Geometry: final body of the model. Coordinates: model frame, mm. Give positions to 0.01 mm unless a question says otherwise; leave off trailing zeros. Write each loop counter-clockwise with the first axis right and the second up, starting at its lowest first coordinate (ties: lowest second). Pieces come first, ordered by that corner, then holes. Notation, with made-up numbers: M 81,87 L 91,87 A25 cw 91,105 Z; hole C 80.5,88.25 d10. An arc over 180 degrees is marked long. Answer as a JSON object with one key per item and string values.
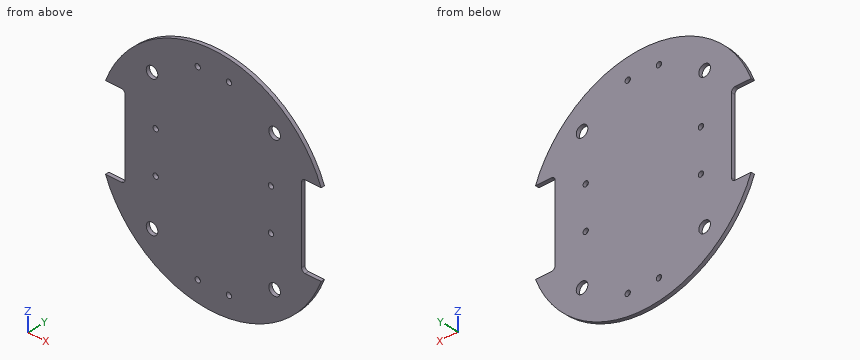
from build123d import *

# Parameters (mm, degrees)
SKETCH1_R               = 49.78
EXTRUDE1_DEPTH          = 1.5875
SKETCH2_R               = 2.5
EXTRUDE2_DEPTH          = 10
CUT_EXTRUDE1_DEPTH      = 71.417447811
FILLET5_R               = 1.6
FILLET5_OF_MIRROR4_R    = 1.6
SKETCH4_R               = 1.145
CUT_EXTRUDE2_DEPTH      = 69.130587523
MIRROR7_COPY_1_SKETCH_R = 1.145
MIRROR7_COPY_1_DEPTH    = 69.130587523
SKETCH6_R               = 1.143
CUT_EXTRUDE4_DEPTH      = 69.130587523
MIRROR9_COPY_1_SKETCH_R = 1.143
MIRROR9_COPY_1_DEPTH    = 69.130587523


with BuildPart() as part:
    # Sketch1 → Extrude1 (new body)
    with BuildSketch(Plane(origin=(0, 0, 0), x_dir=(1, 0, 0), z_dir=(0, 1, 0))):
        with Locations(Location((0, 0, 0), (0, 0, 270))):
            Circle(SKETCH1_R)
    extrude(amount=EXTRUDE1_DEPTH)

    # Sketch2 → Extrude2 (cut)
    with BuildSketch(Plane(origin=(0, 1.5875, 0), x_dir=(-1, 0, 0), z_dir=(0, 1, 0))):
        with Locations(Location((-26.42, -29.72, 0), (0, 0, 90))):
            Circle(SKETCH2_R)
        with Locations(Location((-26.42, 29.72, 0), (0, 0, 90))):
            Circle(SKETCH2_R)
    extrude2 = extrude(amount=-EXTRUDE2_DEPTH, mode=Mode.SUBTRACT)

    # Sketch3 → Cut-Extrude1 (cut, through all)
    with BuildSketch(Plane(origin=(0, 1.5875, 0), x_dir=(1, 0, 0), z_dir=(0, 1, 0))):
        with BuildLine():
            Line((38.03, 0), (38.03, 17.8))
            Line((38.03, 17.8), (46.488798651, 17.8))
            ThreePointArc((46.488798651, 17.8), (49.78, 0), (46.488798651, -17.8))
            Line((46.488798651, -17.8), (38.03, -17.8))
            Line((38.03, -17.8), (38.03, 0))
        make_face()
    cut_extrude1 = extrude(amount=-CUT_EXTRUDE1_DEPTH, mode=Mode.SUBTRACT)

    # Fillet5
    fillet5_edges = [part.edges().sort_by_distance(p)[0] for p in [
        (38.03, 0.79375, 17.8),
        (38.03, 0.79375, -17.8),
    ]]
    fillet(fillet5_edges, radius=FILLET5_R)

    # Mirror4: Cut-Extrude1 across plane
    add(cut_extrude1.mirror(Plane(origin=(0, 0, 0), x_dir=(0, 0, 1), z_dir=(1, 0, 0))), mode=Mode.SUBTRACT)

    # Fillet5 of Mirror4
    fillet5_of_mirror4_edges = [part.edges().sort_by_distance(p)[0] for p in [
        (-38.03, 0.79375, 17.8),
        (-38.03, 0.79375, -17.8),
    ]]
    fillet(fillet5_of_mirror4_edges, radius=FILLET5_OF_MIRROR4_R)

    # Sketch4 → Cut-Extrude2 (cut, through all)
    with BuildSketch(Plane(origin=(0, 1.5875, 0), x_dir=(1, 0, 0), z_dir=(0, 1, 0))):
        with Locations(Location((6.73, 40.5, 0), (0, 0, 270))):
            Circle(SKETCH4_R)
    cut_extrude2 = extrude(amount=-CUT_EXTRUDE2_DEPTH, mode=Mode.SUBTRACT)

    # Mirror5: Cut-Extrude2 across plane
    add(cut_extrude2.mirror(Plane(origin=(0, 0, 0), x_dir=(0, 0, 1), z_dir=(1, 0, 0))), mode=Mode.SUBTRACT)

    # Mirror7: Cut-Extrude2 across plane
    add(cut_extrude2.mirror(Plane.XY), mode=Mode.SUBTRACT)

    # Mirror7 copy 1 sketch → Mirror7 copy 1 (cut, through all)
    with BuildSketch(Plane(origin=(0, 1.5875, 0), x_dir=(-1, 0, 0), z_dir=(0, 1, 0))):
        with Locations(Location((6.73, 40.5, 0), (0, 0, 270))):
            Circle(MIRROR7_COPY_1_SKETCH_R)
    extrude(amount=-MIRROR7_COPY_1_DEPTH, mode=Mode.SUBTRACT)

    # Mirror1: Extrude2 across plane
    add(extrude2.mirror(Plane(origin=(0, 0, 0), x_dir=(0, 0, 1), z_dir=(1, 0, 0))), mode=Mode.SUBTRACT)

    # Sketch6 → Cut-Extrude4 (cut, through all)
    with BuildSketch(Plane(origin=(0, 1.5875, 0), x_dir=(1, 0, 0), z_dir=(0, 1, 0))):
        with Locations(Location((24.83, 9, 0), (0, 0, 270))):
            Circle(SKETCH6_R)
    cut_extrude4 = extrude(amount=-CUT_EXTRUDE4_DEPTH, mode=Mode.SUBTRACT)

    # Mirror8: Cut-Extrude4 across plane
    add(cut_extrude4.mirror(Plane.XY), mode=Mode.SUBTRACT)

    # Mirror9: Cut-Extrude4 across plane
    add(cut_extrude4.mirror(Plane(origin=(0, 0, 0), x_dir=(0, 0, 1), z_dir=(1, 0, 0))), mode=Mode.SUBTRACT)

    # Mirror9 copy 1 sketch → Mirror9 copy 1 (cut, through all)
    with BuildSketch(Plane(origin=(0, 1.5875, 0), x_dir=(-1, 0, 0), z_dir=(0, 1, 0))):
        with Locations(Location((24.83, 9, 0), (0, 0, 270))):
            Circle(MIRROR9_COPY_1_SKETCH_R)
    extrude(amount=-MIRROR9_COPY_1_DEPTH, mode=Mode.SUBTRACT)


solid = part.part
1) Line query: line 1 (X direction, y = 0.5, z = -40.5) (3 decimals); line 2 (X direction, y = 1.5, z = 39.5); line 3 (Z direction, x = -24.83, y = 1.1). Output: solid intervals per line, ascending. Write a range as from..to.
Geometry check:
{"line 1": "x = -28.945..-7.875, -5.585..5.585, 7.875..28.945", "line 2": "x = -30.3..-7.29, -6.17..6.17, 7.29..30.3", "line 3": "z = -43.15..-31.65, -27.79..-10.14, -7.86..7.86, 10.14..27.79, 31.65..43.15"}
2) Contact query for a flat-ended pin moving along its axis: P1, Ø6, axis at x = -26.42, z = 29.72, coming from the -Y side. Output: stop coordinate, or through.
Geometry check:
{"P1": "stops at y = 0"}
3) Cut plane D-D on z = -2. Return loops of the section in (x, y).
Geometry check:
{"outline": "M -38.03,0 L 38.03,0 L 38.03,1.59 L -38.03,1.59 Z"}
4) Cut plane C-C on x = 6.73. Return loops of the section in (y, z) (1 decimal).
Geometry check:
{"outline": "M 0,-49.3 L 1.6,-49.3 L 1.6,-41.6 L 0,-41.6 Z; M 0,-39.4 L 1.6,-39.4 L 1.6,39.4 L 0,39.4 Z; M 0,41.6 L 1.6,41.6 L 1.6,49.3 L 0,49.3 Z"}
5) Cut plane B-B on z = -29.72. Return loops of the section in (x, y), and give its area (3 significant figures).
Geometry check:
{"outline": "M -39.93,0 L -28.92,0 L -28.92,1.59 L -39.93,1.59 Z; M -23.92,0 L 23.92,0 L 23.92,1.59 L -23.92,1.59 Z; M 28.92,0 L 39.93,0 L 39.93,1.59 L 28.92,1.59 Z", "area": "111 mm2"}
6) Cut plane A-A on y = 0.45. Give the number of separate pieces and of enclosed holes in the cut face, and give its area (3 significant figures).
Geometry check:
{"separate pieces": "1", "enclosed holes": "12", "area": "6,920 mm2"}
